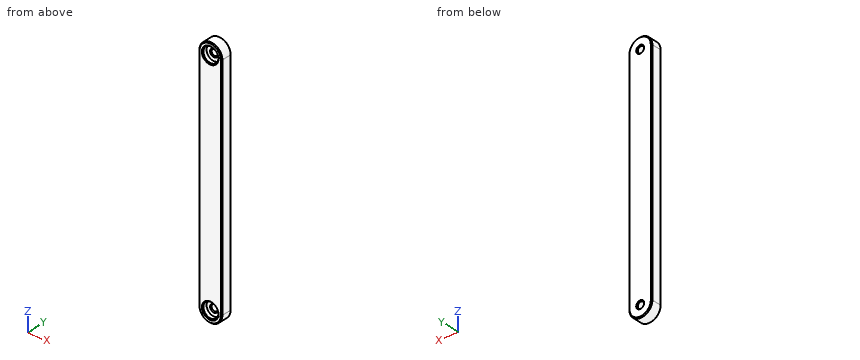
```python
from build123d import *

# Parameters (mm, degrees)
SKETCH1_R           = 2.7
BOSS_EXTRUDE1_DEPTH = 10
SKETCH2_R           = 6.5
CUT_EXTRUDE1_DEPTH  = 4
CHAMFER1_SIZE       = 0.75


with BuildPart() as part:
    # Sketch1 → Boss-Extrude1 (new body)
    with BuildSketch(Plane(origin=(0, 0, 0), x_dir=(1, 0, 0), z_dir=(0, 1, 0))):
        with BuildLine():
            Line((10, -100), (10, 100))
            ThreePointArc((10, 100), (0, 110), (-10, 100))
            Line((-10, 100), (-10, -100))
            ThreePointArc((-10, -100), (0, -110), (10, -100))
        make_face()
        with Locations(Location((0, -100, 0), (0, 0, 270))):
            Circle(SKETCH1_R, mode=Mode.SUBTRACT)
        with Locations(Location((0, 100, 0), (0, 0, 270))):
            Circle(SKETCH1_R, mode=Mode.SUBTRACT)
    extrude(amount=BOSS_EXTRUDE1_DEPTH)

    # Sketch2 → Cut-Extrude1 (cut)
    with BuildSketch(Plane.XZ):
        with Locations(Location((0, 100, 0), (0, 0, 270))):
            Circle(SKETCH2_R)
        with Locations(Location((0, -100, 0), (0, 0, 270))):
            Circle(SKETCH2_R)
    extrude(amount=-CUT_EXTRUDE1_DEPTH, mode=Mode.SUBTRACT)

    # Chamfer1
    chamfer1_edges = [part.edges().sort_by_distance(p)[0] for p in [
        (0, 10, 97.3),
        (10, 10, 0),
        (0, 10, -110),
        (0, 4, 97.3),
        (0, 0, 106.5),
        (0, 0, -93.5),
        (0, 4, -102.7),
        (-10, 10, 0),
        (0, 10, 110),
        (0, 10, -102.7),
        (0, 0, 110),
        (-10, 0, 0),
        (0, 0, -110),
        (10, 0, 0),
    ]]
    chamfer(chamfer1_edges, length=CHAMFER1_SIZE)


solid = part.part
```
Build history of the part. All positions in model axes, mm. Round coordinates to 2 decimals unless told otherwise and drop trailing zeros. Write each loop counter-clockwise with the first axis right and the second up, starting at its lowest first coordinate (ties: lowest second). Pieces come first, ordered by that corner, then holes.
1) Band-saw the part on B-B, the plane x = 0. Give the number of separate pieces and of enclosed holes in the cut face, and give its area (3 significant figures).
2) Drill centre lines: probe 1 along Z at (x, y) = (0, 7.45); probe 2 along Z at (x, y) = (-2.5, 4.5); probe 3 along X at (y, z) = (2.75, 100). Where is each one in solid material? Low to high.
3) Pin check, flat tips, straight feed: pin 1 (7 mm diameter, centred on x = 0, z = 100, fed in from -Y); pin 2 (6 mm diameter, centred on x = 0, z = -100, fed in from +Y). Stop position of each tip, or through.
4) Band-saw the part on A-A, the plane y = 2.5. List the corners of the cut face in (x, z), and give its area (3 significant figures).
Ans:
1. separate pieces: 3
1. enclosed holes: 0
1. area: 2,030 mm2
2. probe 1: z = -110 to -102.7, -97.3 to 97.3, 102.7 to 110
2. probe 2: z = -109.68 to -101.57, -98.43 to 98.43, 101.57 to 109.68
2. probe 3: x = -10 to -6.5, 6.5 to 10
3. pin 1: stops at y = 4
3. pin 2: stops at y = 9.55
4. outline: (-10, -100) arc R10 ccw to (10, -100) - (10, 100) arc R10 ccw to (-10, 100) - close; hole circle Ø13 at (0, -100); hole circle Ø13 at (0, 100)
4. area: 4,050 mm2
